from build123d import *

# Parameters (mm, degrees)
F1_DEPTH = 63.5
F2_DEPTH = 25.4
F3_DEPTH = 7.9375
F0_W     = 24.147347727
F0_H     = 19.05
F4_DEPTH = 25.4
F6_R     = 6.35


with BuildPart() as f1:
    # F0 (on Front) → F1 (new body, symmetric)
    with BuildSketch(Plane.XZ):
        Polygon((-41.275, 9.525), (-41.275, -9.525), (41.275, -9.525), (41.275, 9.525), (22.225, 9.525), align=None)
    extrude(amount=F1_DEPTH, both=True)

    # F0 (on Front) → F2 (join, symmetric)
    with BuildSketch(Plane.XZ):
        with BuildLine():
            Line((22.225, 9.525), (41.275, 9.525))
            Line((41.275, 9.525), (41.275, 28.2702))
            ThreePointArc((41.275, 28.2702), (45.9246798487, 39.4955201513), (57.15, 44.1452))
            Line((57.15, 44.1452), (60.325, 44.1452))
            Line((60.325, 44.1452), (60.325, 63.1952))
            Line((60.325, 63.1952), (57.15, 63.1952))
            ThreePointArc((57.15, 63.1952), (32.4542956671, 52.9659043329), (22.225, 28.2702))
            Line((22.225, 28.2702), (22.225, 9.525))
        make_face()
    extrude(amount=F2_DEPTH, both=True)

    # F0 (on Front) → F3 (join, symmetric)
    with BuildSketch(Plane.XZ):
        with BuildLine():
            add(Edge.make_bspline(
                [(57.15, 63.1952), (12.8750428557, 65.7868459821), (-41.9757738709, 38.8200096786), (-41.275, 9.525)],
                knots=[0, 0, 0, 0, 112.1069622862, 112.1069622862, 112.1069622862, 112.1069622862], degree=3))
            Line((-41.275, 9.525), (22.225, 9.525))
            Line((22.225, 9.525), (22.225, 28.2702))
            ThreePointArc((22.225, 28.2702), (32.4542956671, 52.9659043329), (57.15, 63.1952))
        make_face()
    extrude(amount=F3_DEPTH, both=True)

    # F0 (on Front) → F4 (join, symmetric)
    with BuildSketch(Plane.XZ):
        with Locations((72.3986738635, 53.6702)):
            Rectangle(F0_W, F0_H)
    extrude(amount=F4_DEPTH, both=True)

    # F0 (on Front) → F5 (revolve)
    with BuildSketch(Plane.XZ):
        Polygon((84.472347727, 66.675), (84.472347727, 63.1952), (84.472347727, 44.1452), (84.472347727, 38.1), (111.125, 38.1), (111.125, 66.675), align=None)
    revolve(axis=Axis((84.472347727, 0, 52.3875), (0, 0, -1)))

    # F6
    f6_edges = [f1.edges().sort_by_distance(p)[0] for p in [
        (-41.275, -63.5, 0),
        (41.275, -63.5, 0),
        (-41.275, 63.5, 0),
        (41.275, 63.5, 0),
    ]]
    fillet(f6_edges, radius=F6_R)


solid = f1.part
The listing builds one solid part. Answer for the finished solid, in the listing's coordinates (mm). A direction names the side the tool comes from. Round coordinates to 2 decimals unless told otherwise and drop trailing zeros. Write each loop counter-clockwise with the first axis right and the second up, starting at its lowest first coordinate (ties: lowest second). Pieces come first, ordered by that corner, then holes. Notation, with made-up numbers: M -19.5,-14.75 L 8.5,-14.75 A30 ccw 8.5,22.25 Z; hole C -8,55 d9. An arc over 180 degrees is marked long. Write each question's results on one line, items separated by ' | '. Start each with the question number.
Item 1: Straight lines are drawn through the part: probe 1 along X at (y, z) = (38, -2.5) (3 decimals); probe 2 along Z at (x, y) = (72, 14) (3 decimals); probe 3 along Y at (x, z) = (-24, 36.5). For each, find the intervals that lie inside material, in ascending order.
Item 2: Given pin 1 Ø3 at (x, z) = (6, 31) entering from +Y; pin 2 Ø16 at (x, z) = (57.5, 37) entering from +Y; pin 3 Ø21 at (x, y) = (68, 0) entering from -Z, each flat-ended and moving along its own axis, determine where each tip first touches the part or whether it passes through.
Item 3: Which of the six approach directions +Z, -Z, +X, -X, +Y, -Y give full straight-line access (tool end or side, diameter ignored) to faces 1 (the flat face through (57.5, -2, 44.145)), 2 (the flat face through (-4, -7.938, 32)), 3 (the flat face through (85, 0, 38.1))?
Item 4: Find section B-B on y = -10. Write down the section's boundary in (x, z) (3 decimals).
Item 5: Find section A-A on z = 5. Write down the section's boundary in (x, y) (3 decimals).
Item 6: Find section C-C on y = -37. Write down the section's boundary in (x, z) (3 decimals), and give its area (3 significant figures).
Answer block:
1) probe 1: x = -41.275 to 41.275 | probe 2: z = 38.1 to 66.675 | probe 3: y = -7.94 to 7.94
2) pin 1: stops at y = 7.94 | pin 2: stops at y = 25.4 | pin 3: stops at z = 38.1
3) face 1: -Z | face 2: +Z, -X, -Y | face 3: -Z, +X, +Y, -Y
4) outline: M -41.275,-9.525 L 41.275,-9.525 L 41.275,28.27 A15.875 cw 57.15,44.145 L 59.767,44.145 L 59.767,38.1 L 109.178,38.1 L 109.178,66.675 L 59.767,66.675 L 59.767,63.195 L 57.15,63.195 A34.925 ccw 22.225,28.27 L 22.225,9.525 L -41.275,9.525 Z
5) outline: M -41.275,-57.15 A6.35 ccw -34.925,-63.5 L 34.925,-63.5 A6.35 ccw 41.275,-57.15 L 41.275,57.15 A6.35 ccw 34.925,63.5 L -34.925,63.5 A6.35 ccw -41.275,57.15 Z
6) outline: M -41.275,-9.525 L 41.275,-9.525 L 41.275,9.525 L -41.275,9.525 Z | area: 1,570 mm²
